Check sheet for the modelled part. Datum: model origin and axes. Units: mm. Face numbers are marked on the shaded views. A direction names the side the tool comes from. Round coordinates to 2 decimals unless told otherwise and drop trailing zeros. Write each loop counter-clockwise with the first axis right and the second up, starting at its lowest first coordinate (ties: lowest second). Pieces come first, ordered by that corner, then holes. Notation, with made-up numbers: M 8,-40 L 51,-40 A16 cw 51,-13 Z; hole C 47,43 d5. An arc over 180 degrees is marked long. One line per item, written item: value.
from build123d import *

# Parameters (mm, degrees)
BOSS_EXTRUDE1_START = 3.5
SKETCH1_R           = 1
BOSS_EXTRUDE1_DEPTH = 1
SKETCH2_R           = 1
BOSS_EXTRUDE2_DEPTH = 4.75


with BuildPart() as part:
    # Sketch1 → Boss-Extrude1 (new body)
    with BuildSketch(Plane.YZ.offset(BOSS_EXTRUDE1_START)):
        with BuildLine():
            ThreePointArc((-2.752777778, 3.339194107), (-8.955, 0), (-2.752777778, -3.339194107))
            ThreePointArc((-2.752777778, -3.339194107), (0, -2.513186741), (2.752777778, -3.339194107))
            ThreePointArc((2.752777778, -3.339194107), (8.955, 0), (2.752777778, 3.339194107))
            ThreePointArc((2.752777778, 3.339194107), (0, 2.513186741), (-2.752777778, 3.339194107))
        make_face()
        with Locations(Location((-4.955, 0, 0), (0, 0, 270))):
            Circle(SKETCH1_R, mode=Mode.SUBTRACT)
        with Locations(Location((4.955, 0, 0), (0, 0, 90))):
            Circle(SKETCH1_R, mode=Mode.SUBTRACT)
    extrude(amount=BOSS_EXTRUDE1_DEPTH)


with BuildPart() as body_2:
    # Mirror2: mirrored copy
    add(part.part.mirror(Plane(origin=(0, 0, 0), x_dir=(0, 0, 1), z_dir=(1, 0, 0))))


with BuildPart() as part_1:
    add(part.part)

    add(body_2.part)  # Boss-Extrude2 merges body 2
    # Sketch2 → Boss-Extrude2 (add, symmetric)
    with BuildSketch(Plane.YZ):
        with Locations(Location((-4.955, 0, 0), (0, 0, 90))):
            Circle(SKETCH2_R)
        with Locations(Location((4.955, 0, 0), (0, 0, 90))):
            Circle(SKETCH2_R)
    extrude(amount=BOSS_EXTRUDE2_DEPTH, both=True)


solid = part_1.part
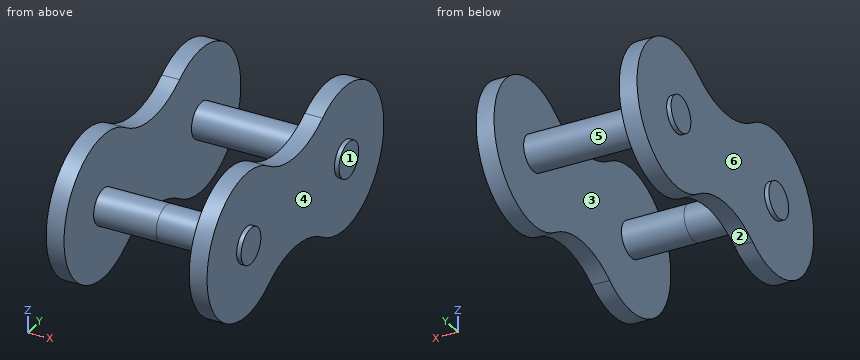
Q1. Sectioned sample at D-D on z = -3. Enter the section's corners in (x, y).
Completed:
outline: M -4.5,-7.6 L -3.5,-7.6 L -3.5,-2.15 L -4.5,-2.15 Z; M -4.5,2.15 L -3.5,2.15 L -3.5,7.6 L -4.5,7.6 Z; M 3.5,-7.6 L 4.5,-7.6 L 4.5,-2.15 L 3.5,-2.15 Z; M 3.5,2.15 L 4.5,2.15 L 4.5,7.6 L 3.5,7.6 Z
Q2. Draft check along X on the marked faces 1, 2 and 3. Enter one of: pulls with the +X half, pulls with the -X half, needs draft (parallel to the pull), parting line crosses it, or undercut.
Completed:
face 1: pulls with the +X half
face 2: needs draft
face 3: undercut
Q3. Scan lines: line 1 (X direction, y = 6, z = 1.75); line 2 (Y direction, x = 1.5, z = 0) (3 decimals); line 3 (Z direction, x = 0, y = 5). Record each from-to range of solid material in increasing order. Write a range as [from, to].
Completed:
line 1: [-4.5, -3.5], [3.5, 4.5]
line 2: [-5.955, -3.955], [3.955, 5.955]
line 3: [-1, 1]
Q4. Access from +Z, -Z, +X, -X, +Y, -Y to the whole of each face (thin tool, end or side, straight path). Record for the marked faces 4, 5 and 6.
Completed:
face 4: +X
face 5: none
face 6: -X
Q5. Depth check by flat-ended pin: P1, Ø2, axis at y = -2, z = -1, coming from the +X side; P2, Ø1.5, axis at x = 3, y = 6, coming from the -Z side; P3, Ø3, axis at x = -3.5, y = -2.5, coming from the +Z side. Enter the tip coordinate at first touch or a pass-through.
Completed:
P1: x = 4.5
P2: z = -3.97
P3: z = 3.88
Q6. Sectioned sample at C-C on z = 1.25. Enter the section's corners in (x, y).
Completed:
outline: M -4.5,-8.75 L -3.5,-8.75 L -3.5,8.75 L -4.5,8.75 Z; M 3.5,-8.75 L 4.5,-8.75 L 4.5,8.75 L 3.5,8.75 Z
Q7. Sectioned sample at B-B on y = 7.75. Enter the section's corners in (x, z).
Completed:
outline: M -4.5,-2.86 L -3.5,-2.86 L -3.5,2.86 L -4.5,2.86 Z; M 3.5,-2.86 L 4.5,-2.86 L 4.5,2.86 L 3.5,2.86 Z
